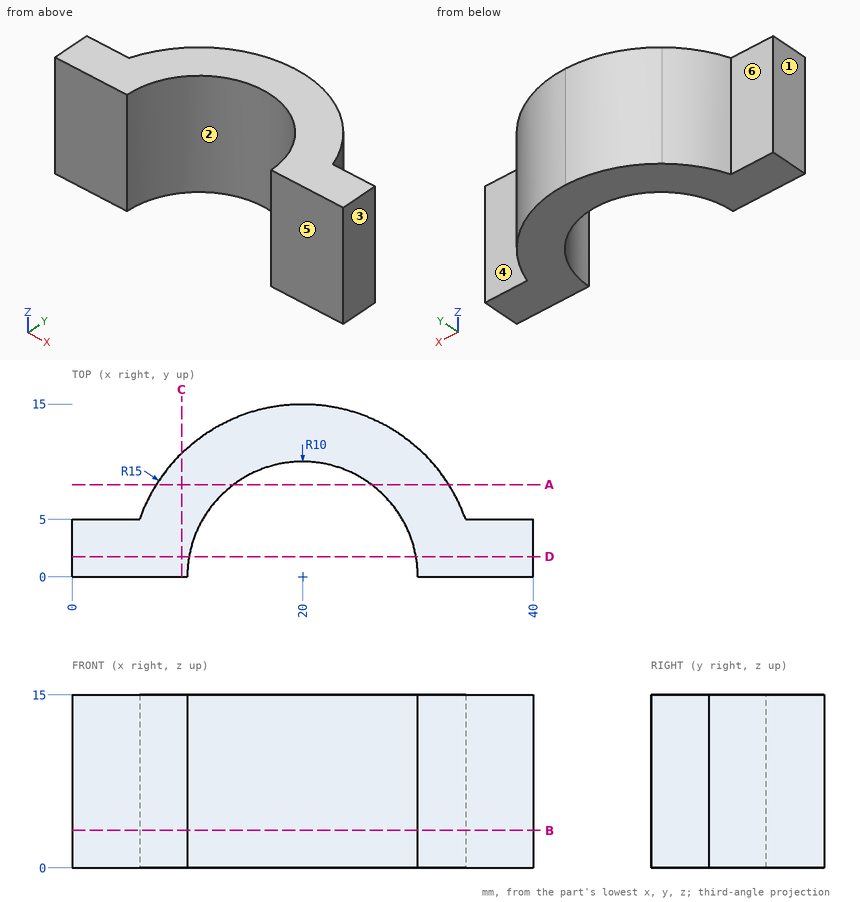
Answer from the drawing. Dimensions are ordinates in mm from the lowest x, y and z of the part. A direction names the side the tool comes from. Round coordinates to 2 decimals unless told otherwise and drop trailing zeros. Loops run counter-clockwise (first coordinate to the right, second up) from the corner with the lowest first, then second, coordinate; pieces in that order, holes last. Notation, with made-up numbers: (16, 33) - (66, 33) arc R28 ccw to (66, 69) - close; hole circle Ø5 at (84.5, -8.5). An arc over 180 degrees is marked (long way). Return JSON: item names as keys, results as strings. Group by question number.
1. The part is cut by section A-A on y = 8. Determine the outline of the cut face in (x, z).
2. Each of these flat-tipped pins is pushed along its axis until it touches: P1, Ø1.5, axis at x = 24.5, y = 8, coming from the +Z side; P2, Ø2, axis at x = 13, z = 7.5, coming from the -Y side; P3, Ø6, axis at y = 9, z = 13, coming from the +X side; P4, Ø8, axis at y = 12.5, z = 5, coming from the -X side. Where does it stop, or does it pass through?
3. The part is cut by section D-D on y = 1.75. Determine the outline of the cut face in (x, z).
4. Consider probe 1 along X at (y, z) = (8.25, 7.25); probe 2 along X at (y, z) = (3.5, 13.75); probe 3 along Y at (x, z) = (35, 3). Determine where each line is inside the solid, lowest interval first.
5. The part is cut by section C-C on x = 9.5. Determine the outline of the cut face in (y, z).
6. The part is cut by section B-B on z = 3.25. Determine the outline of the cut face in (x, y).
7. The mould has two halves that part along X. Classify the marked faces 1, 2, 3 and 4: pulls with the +X half, pulls with the -X half, needs draft (parallel to the pull), parting line crosses it, or undercut.
8. Which of the six approach directions +Z, -Z, +X, -X, +Y, -Y give full straight-line access (tool end or side, diameter ignored) to the marked faces 5 and 6?
Resolved:
{
 "1": {"outline": "(7.31, 0) - (14, 0) - (14, 15) - (7.31, 15) - close; (26, 0) - (32.69, 0) - (32.69, 15) - (26, 15) - close"},
 "2": {"P1": "passes through", "P2": "stops at y = 6", "P3": "stops at x = 33.75", "P4": "stops at x = 7.64"},
 "3": {"outline": "(0, 0) - (10.15, 0) - (10.15, 15) - (0, 15) - close; (29.85, 0) - (40, 0) - (40, 15) - (29.85, 15) - close"},
 "4": {"probe 1": "x = 7.47 to 14.35, 25.65 to 32.53", "probe 2": "x = 0 to 10.63, 29.37 to 40", "probe 3": "y = 0 to 5"},
 "5": {"outline": "(0, 0) - (10.71, 0) - (10.71, 15) - (0, 15) - close"},
 "6": {"outline": "(0, 0) - (10, 0) arc R10 cw to (30, 0) - (40, 0) - (40, 5) - (34.14, 5) arc R15 ccw to (5.86, 5) - (0, 5) - close"},
 "7": {"face 1": "pulls with the -X half", "face 2": "undercut", "face 3": "pulls with the +X half", "face 4": "needs draft"},
 "8": {"face 5": "+Z, -Z, +X, -X, -Y", "face 6": "+Z, -Z, -X, +Y"}
}
